Geometry check sheet. Reference: drawing and pictorial views, mm from the part's lowest x, y, z. A direction names the side the tool comes from. Give positions to 0.01 mm unless a question says otherwise; leave off trailing zeros. Write each loop counter-clockwise with the first axis right and the second up, starting at its lowest first coordinate (ties: lowest second). Pieces come first, ordered by that corner, then holes. Notation, with made-up numbers: (-33.5, 11) -> (5.5, 11) arc R26 ccw to (5.5, 43) -> close; hole circle Ø3 at (-38.75, 74). An arc over 180 degrees is marked (long way). Return JSON: item names as keys, results as strings.
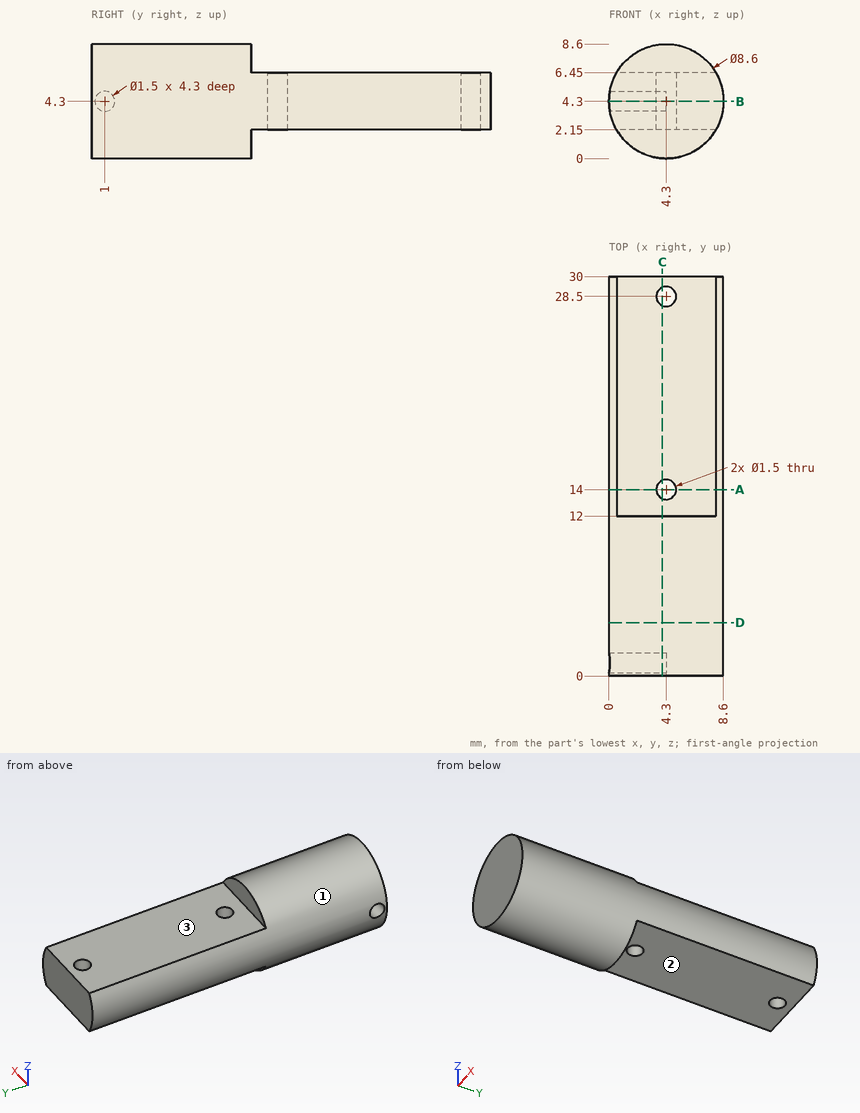
(1) Set-up check for the marked faces 1, 2 and 3: record each of +Z, -Z, +X, -X, +Y, -Y from which the full face is reachable in a straight line by a thin tool's end or side.
Reply:
{"face 1": "+Y, -Y", "face 2": "-Z, +X, -X, +Y", "face 3": "+Z, +X, -X, +Y"}
(2) Cross-section at C-C on x = 4. Enter the section's corners in (y, z), then the cut area to 3 significant figures.
Reply:
{"outline": "(0, 0.01) -> (12, 0.01) -> (12, 2.15) -> (13.31, 2.15) -> (13.31, 6.45) -> (12, 6.45) -> (12, 8.59) -> (0, 8.59) -> close; (14.69, 2.15) -> (27.81, 2.15) -> (27.81, 6.45) -> (14.69, 6.45) -> close; (29.19, 2.15) -> (30, 2.15) -> (30, 6.45) -> (29.19, 6.45) -> close; hole circle Ø1.5 at (1, 4.3)", "area": "167 mm^2"}
(3) Depth check by flat-ended pin: pin 1 Ø2 at (x, y) = (4.5, 23) entering from -Z; pin 2 Ø1 at (x, y) = (2, 10.5) entering from -Z; pin 3 Ø1.5 at (y, z) = (18.5, 5.5) entering from +X. Enter the tip coordinate at first touch or a pass-through.
Reply:
{"pin 1": "z = 2.15", "pin 2": "z = 0.39", "pin 3": "x = 8.58"}
(4) Thickness scan on L1, parallel to Y at x = 4.3, z = 3.3; L2, parallel to Y at x = 1.2, z = 4.3; L3, parallel to Z at x = 2.25, y = 25. Record the ranges inside material, lowest first.
Reply:
{"L1": "0 to 13.25, 14.75 to 27.75, 29.25 to 30", "L2": "0 to 0.25, 1.75 to 30", "L3": "2.15 to 6.45"}
(5) Cross-section at A-A on y = 14. Enter the section's corners in (x, z).
Reply:
{"outline": "(0.58, 2.15) -> (3.55, 2.15) -> (3.55, 6.45) -> (0.58, 6.45) arc R4.3 ccw to start; (5.05, 2.15) -> (8.02, 2.15) arc R4.3 ccw to (8.02, 6.45) -> (5.05, 6.45) -> close"}
(6) Cross-section at D-D on y = 4. Enter the section's corners in (x, z), then the cut area to 3 significant figures.
Reply:
{"outline": "circle Ø8.6 at (4.3, 4.3)", "area": "58.1 mm^2"}
(7) Cross-section at B-B on z = 4.3. Enter the section's corners in (x, y).
Reply:
{"outline": "(0, 0) -> (8.6, 0) -> (8.6, 30) -> (0, 30) -> (0, 1.75) -> (4.3, 1.75) -> (4.3, 0.25) -> (0, 0.25) -> close; hole circle Ø1.5 at (4.3, 14); hole circle Ø1.5 at (4.3, 28.5)"}
